Design review of the part built by this model. Coordinates are the model's own, in mm. A direction names the side the tool comes from. Give positions to 0.01 mm unless a question says otherwise; leave off trailing zeros. Order: outer loops, then holes, each group sorted by start corner. A loop starts at its lowest first (then second) coordinate and runs counter-clockwise, first axis right, second up. Notation, with made-up numbers: (86, 38.25) -> (143, 38.25) arc R24 cw to (143, 68.25) -> close; hole circle Ø2 at (36, 40.25). An arc over 180 degrees is marked (long way). Use a Markdown table: item, result. Add a question column.
```python
from build123d import *

# Parameters (mm, degrees)
ESQUISSE1_W             = 32.21
ESQUISSE1_H             = 20.49
ESQUISSE1_R             = 1.5
BOSS_EXTRU_1_DEPTH      = 2
ESQUISSE2_W             = 4
ESQUISSE2_H             = 10.471151719
BOSS_EXTRU_2_DEPTH      = 10
ESQUISSE3_R             = 1.75
ENL_V_MAT_EXTRU_1_DEPTH = 10


with BuildPart() as part:
    # Esquisse1 → Boss.-Extru.1 (new body)
    with BuildSketch(Plane.XY):
        with Locations((16.105, 10.245)):
            Rectangle(ESQUISSE1_W, ESQUISSE1_H)
        with Locations((27.21, 15.49)):
            Circle(ESQUISSE1_R, mode=Mode.SUBTRACT)
        with Locations((5, 5)):
            Circle(ESQUISSE1_R, mode=Mode.SUBTRACT)
    extrude(amount=BOSS_EXTRU_1_DEPTH)

    # Esquisse2 → Boss.-Extru.2 (add)
    with BuildSketch(Plane.XY.offset(2)):
        with Locations((22, 10.23557586)):
            Rectangle(ESQUISSE2_W, ESQUISSE2_H)
    extrude(amount=BOSS_EXTRU_2_DEPTH)

    # Esquisse3 → Enlèv. mat.-Extru.1 (cut)
    with BuildSketch(Plane(origin=(24, 0, 0), x_dir=(0, 0, -1), z_dir=(1, 0, 0))):
        with Locations((-7.092486799, 13.5)):
            Circle(ESQUISSE3_R)
        with Locations((-7.092486799, 7.5)):
            Circle(ESQUISSE3_R)
    extrude(amount=-ENL_V_MAT_EXTRU_1_DEPTH, mode=Mode.SUBTRACT)


solid = part.part
```
1) Add section D-D (y = 10). Give the boundary of the cut face in (x, z).
2) The part is to be moulded in two halves that separate along Y. For faces 6 (the cylindrical face through (25.71, 15.56, 0.99)), 7 (the flat face through (32.21, 10, 1)), 8 (the flat face through (16, 20.49, 1)), 9 (the flat face through (22, 5, 7)), say which applies: +Y half, -Y half, draft (parallel to the pull), parting line (faces both ways), or undercut.
3) Insertion check: pin 1 (4 mm diameter, centred on y = 7.5, z = 7.09, fed in from -X); pin 2 (2 mm diameter, centred on x = 21, z = 9, fed in from +Y); pin 3 (6 mm diameter, centred on x = 6.5, y = 15, fed in from +Z); pin 4 (6 mm diameter, centred on x = 10.5, y = 15, fed in from -Z). Each pin has a flat end and moves straight along its axis. Give the tip position at first contact, or say it passes through.
4) Add section B-B (x = 5). Give the boundary of the cut face in (y, z), then the cut area to 3 significant figures.
5) Add section C-C (z = 6.25). Give the boundary of the cut face in (x, y), then the cut area to 3 significant figures.
6) Add section A-A (y = 13.5). Give the boundary of the cut face in (x, z), then the cut area to 3 significant figures.
7) Machinability: for faces 1 (the flat face through (16, 0, 1)), 2 (the flat face through (16, 10, 0)), 3 (the flat face through (20, 10, 7)), 4 (the flat face through (24, 10, 7)), 5 (the flat face through (22, 15.471, 7)), which of the approach directions +Z, -Z, +X, -X, +Y, -Y give a long, thin tool a straight path to every point of the face, cutting with its end or side? Answer none if there is none.
8) For L1, parallel to Y at x = 27.21, z = 1.1; L2, parallel to Y at x = 5, z = 0.5; L3, parallel to Z at x = 4, y = 13.25, list the stretches that pass through material, from the lowest coordinate up. Write a range as [from, to].
Worked answers:
| question | item | result |
|---|---|---|
| 1 | outline | (0, 0) -> (32.21, 0) -> (32.21, 2) -> (24, 2) -> (24, 12) -> (20, 12) -> (20, 2) -> (0, 2) -> close |
| 2 | face 6 | undercut |
| 2 | face 7 | draft |
| 2 | face 8 | +Y half |
| 2 | face 9 | -Y half |
| 3 | pin 1 | x = 20 |
| 3 | pin 2 | y = 15.47 |
| 3 | pin 3 | z = 2 |
| 3 | pin 4 | z = 0 |
| 4 | outline | (0, 0) -> (3.5, 0) -> (3.5, 2) -> (0, 2) -> close; (6.5, 0) -> (20.49, 0) -> (20.49, 2) -> (6.5, 2) -> close |
| 4 | area | 35.0 mm^2 |
| 5 | outline | (20, 5) -> (24, 5) -> (24, 5.97) -> (20, 5.97) -> close; (20, 9.03) -> (24, 9.03) -> (24, 11.97) -> (20, 11.97) -> close; (20, 15.03) -> (24, 15.03) -> (24, 15.47) -> (20, 15.47) -> close |
| 5 | area | 17.3 mm^2 |
| 6 | outline | (0, 0) -> (32.21, 0) -> (32.21, 2) -> (24, 2) -> (24, 5.34) -> (20, 5.34) -> (20, 2) -> (0, 2) -> close; (20, 8.84) -> (24, 8.84) -> (24, 12) -> (20, 12) -> close |
| 6 | area | 90.4 mm^2 |
| 7 | face 1 | +Z, -Z, +X, -X, -Y |
| 7 | face 2 | -Z, +X, -X, +Y, -Y |
| 7 | face 3 | +Z, -X, +Y, -Y |
| 7 | face 4 | +Z, +X, +Y, -Y |
| 7 | face 5 | +Z, +X, -X, +Y |
| 8 | L1 | [0, 13.99], [16.99, 20.49] |
| 8 | L2 | [0, 3.5], [6.5, 20.49] |
| 8 | L3 | [0, 2] |
